Check sheet for the drawn part. Datum: minimum x, y, z corner. Units: mm. A direction names the side the tool comes from. Round coordinates to 2 decimals unless told otherwise and drop trailing zeros. Loops run counter-clockwise (first coordinate to the right, second up) from the corner with the lowest first, then second, coordinate; pieces in that order, holes last. Notation, with made-up numbers: (43, -6) -> (63, -6) arc R18 cw to (63, 29) -> close; hole circle Ø7 at (77.5, -26). An arc over 180 degrees is marked (long way). Write item = value, one per line. Start each with the question number.
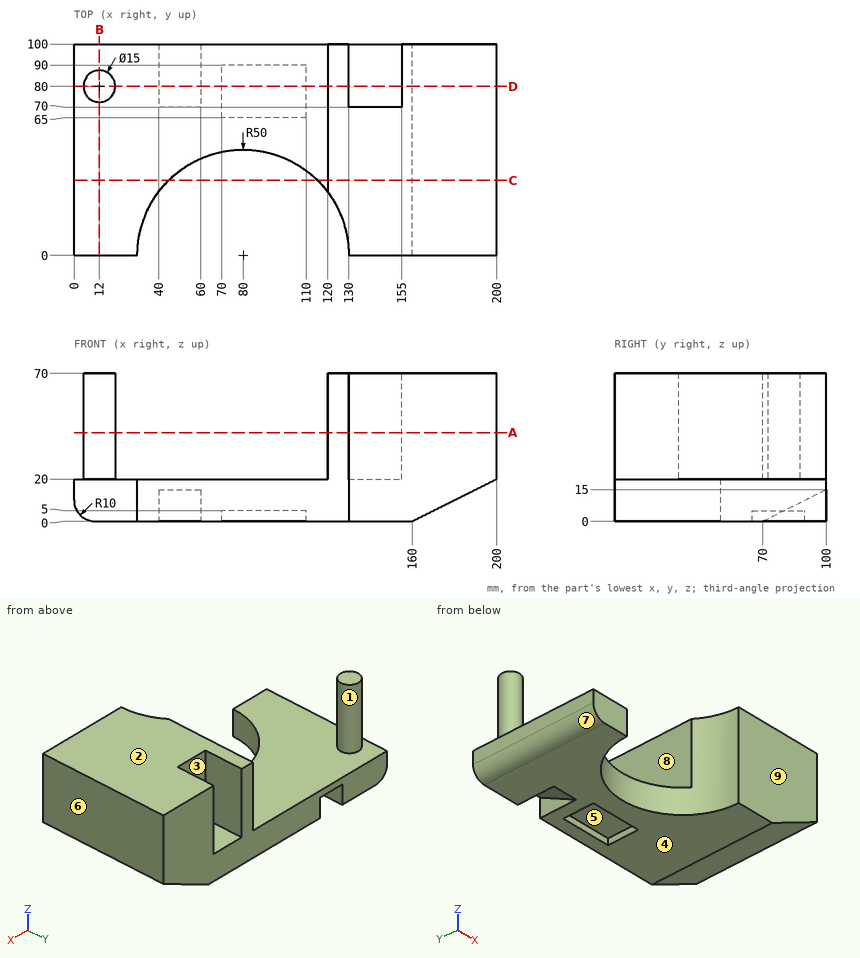
(1) Draft check along X on the marked faces 6, 7, 8 and 9. Enter one of: +X half, -X half, draft (parallel to the pull), parting line (faces both ways), or undercut.
(2) Section check A-A on z = 42. Enter the section's corners in (x, y), then the cut area to 3 significant figures.
(3) Section check B-B on x = 12. Enter the section's corners in (y, z).
(4) Scan lines: line 1 (X direction, y = 74, z = 53.5); line 2 (Y direction, x = 148, z = 30.5); line 3 (X direction, y = 47, z = 27.5). Record each from-to range of solid material in increasing order. Write a range as [from, to].
(5) Section check C-C on y = 35.5. Enter the section's corners in (x, z), then the cut area to 3 significant figures.
(6) Depth check by flat-ended pin: pin 1 Ø7.5 at (y, z) = (84.5, 8.5) entering from +X; pin 2 Ø10 at (y, z) = (70, 57) entering from -X; pin 3 Ø4 at (y, z) = (72, 3) entering from -X. Enter the tip coordinate at first touch or a pass-through.
(7) Section check D-D on y = 80. Enter the section's corners in (x, z), then the cut area to 3 significant figures.
(8) Access from +Z, -Z, +X, -X, +Y, -Y to the whole of each face (thin tool, end or side, straight path). Record for the marked faces 1, 2, 3, 4 and 5.
Computed values:
q1.face_6 = +X half
q1.face_7 = -X half
q1.face_8 = undercut
q1.face_9 = draft
q2.outline = circle Ø15 at (12, 80); (120, 30) arc R50 cw to (130, 0) -> (200, 0) -> (200, 100) -> (155, 100) -> (155, 70) -> (130, 70) -> (130, 100) -> (120, 100) -> close
q2.area = 7,220 mm²
q3.outline = (0, 0) -> (100, 0) -> (100, 20) -> (87.5, 20) -> (87.5, 70) -> (72.5, 70) -> (72.5, 20) -> (0, 20) -> close
q4.line_1 = [7.5, 16.5], [120, 130], [155, 200]
q4.line_2 = [0, 70]
q4.line_3 = [120, 200]
q5.outline = (0, 10) arc R10 ccw to (10, 0) -> (44.79, 0) -> (44.79, 20) -> (0, 20) -> close; (115.21, 0) -> (160, 0) -> (200, 20) -> (200, 70) -> (120, 70) -> (120, 20) -> (115.21, 20) -> close
q5.area = 6,170 mm²
q6.pin_1 = 184.5
q6.pin_2 = 6.41
q6.pin_3 = 1.34
q7.outline = (0, 10) arc R10 ccw to (10, 0) -> (40, 0) -> (40, 5) -> (60, 5) -> (60, 0) -> (70, 0) -> (70, 5) -> (110, 5) -> (110, 0) -> (160, 0) -> (200, 20) -> (200, 70) -> (155, 70) -> (155, 20) -> (130, 20) -> (130, 70) -> (120, 70) -> (120, 20) -> (19.5, 20) -> (19.5, 70) -> (4.5, 70) -> (4.5, 20) -> (0, 20) -> close
q7.area = 6,780 mm²
q8.face_1 = +Z
q8.face_2 = +Z, +X, -X, +Y, -Y
q8.face_3 = +Z, +Y
q8.face_4 = -Z, +X, -X, +Y, -Y
q8.face_5 = -Z
